Job drawing, mm, ordinate dimensions from the low corner. One solid piece. A direction names the side the tool comes from. Give positions to 0.01 mm unless a question says otherwise; leave off trailing zeros. Write each loop counter-clockwise with the first axis right and the second up, starting at its lowest first coordinate (ties: lowest second). Pieces come first, ordered by that corner, then holes. Notation, with made-up numbers: (37, 29.25) -> (53, 29.25) arc R18 cw to (53, 42.25) -> close; hole circle Ø10 at (44, 12.5). An arc over 180 degrees is marked (long way). Put each result on its own line as item: value. Start each with the question number.
Item 1: Tool access for the marked faces 4 and 5: list every direction of +Z, -Z, +X, -X, +Y, -Y with a clear straight run to the whole face (end or side of a thin tool).
Item 2: Slice it at A-A, the plane y = 39.5. List the corners of the cut face in (x, z), plus the area to 3 significant figures.
Item 3: Drill centre lines: line 1 along X through (y, z) = (28.5, 569); line 2 along Z through (x, y) = (327, 24). Where is each one in solid material? Low to high.
Item 4: Slice it at C-C, the plane x = 426.5. List the corners of the cut face in (y, z), plus the area to 3 significant figures.
Item 5: Two-plate mould, pull along X, no slides. Class the marked faces 1, 2 and 3: pulls with the +X half, pulls with the -X half, needs draft (parallel to the pull), parting line crosses it, or undercut.
Item 6: Slice it at B-B, the plane z = 387. List the corners of the cut face in (x, y).
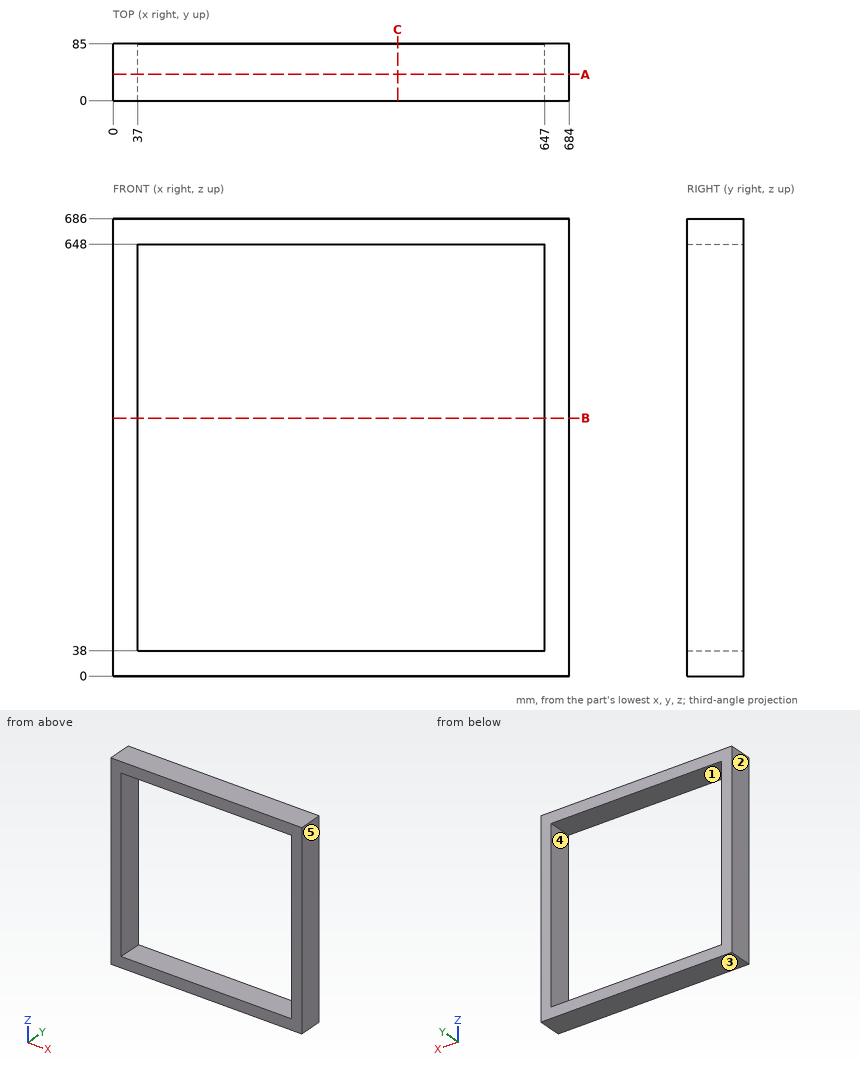
Values follow:
1. face 4: +Y, -Y
1. face 5: +Z, -Z, +X, +Y, -Y
2. outline: (0, 0) -> (684, 0) -> (684, 686) -> (0, 686) -> close; hole (37, 38) -> (647, 38) -> (647, 648) -> (37, 648) -> close
2. area: 97,100 mm2
3. line 1: 0 to 37, 647 to 684
3. line 2: 0 to 38, 648 to 686
4. outline: (0, 0) -> (85, 0) -> (85, 38) -> (0, 38) -> close; (0, 648) -> (85, 648) -> (85, 686) -> (0, 686) -> close
4. area: 6,460 mm2
5. face 1: undercut
5. face 2: pulls with the -X half
5. face 3: needs draft
6. outline: (0, 0) -> (37, 0) -> (37, 85) -> (0, 85) -> close; (647, 0) -> (684, 0) -> (684, 85) -> (647, 85) -> close
